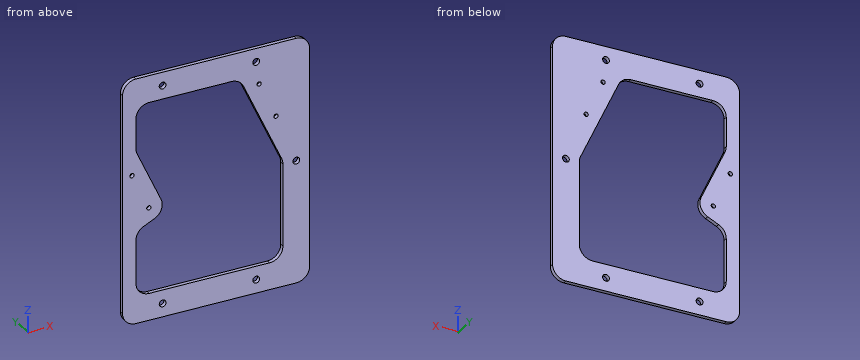
```python
from build123d import *

# Parameters (mm, degrees)
SKETCH_1_W          = 140
SKETCH_1_H          = 182.5
SKETCH_1_R          = 2.55
EXTRUDE_1_DEPTH     = 3
FILLET_1_R          = 10
SKETCH_2_R          = 1.6
CUT_EXTRUDE_1_DEPTH = 116.045914747
CUT_EXTRUDE_2_DEPTH = 116.045914747
FILLET_2_R          = 10


with BuildPart() as part:
    # ｽｹｯﾁ1 → ﾎﾞｽ - 押し出し1 (new body)
    with BuildSketch(Plane(origin=(0, 0, 0), x_dir=(1, 0, 0), z_dir=(0, 1, 0))):
        Rectangle(SKETCH_1_W, SKETCH_1_H)
        with Locations(Location((-40, 81.25, 0), (0, 0, 270))):
            Circle(SKETCH_1_R, mode=Mode.SUBTRACT)
        with Locations(Location((30, 81.25, 0), (0, 0, 270))):
            Circle(SKETCH_1_R, mode=Mode.SUBTRACT)
        with Locations(Location((60, 0, 0), (0, 0, 270))):
            Circle(SKETCH_1_R, mode=Mode.SUBTRACT)
        with Locations(Location((-40, -81.25, 0), (0, 0, 270))):
            Circle(SKETCH_1_R, mode=Mode.SUBTRACT)
        with Locations(Location((30, -81.25, 0), (0, 0, 270))):
            Circle(SKETCH_1_R, mode=Mode.SUBTRACT)
    extrude(amount=EXTRUDE_1_DEPTH)

    # ﾌｨﾚｯﾄ1
    fillet_1_edges = [part.edges().sort_by_distance(p)[0] for p in [
        (70, 1.5, 91.25),
        (-70, 1.5, 91.25),
        (-70, 1.5, -91.25),
        (70, 1.5, -91.25),
    ]]
    fillet(fillet_1_edges, radius=FILLET_1_R)

    # ｽｹｯﾁ2 → ｶｯﾄ - 押し出し1 (cut, through all)
    with BuildSketch(Plane(origin=(0, 3, 0), x_dir=(1, 0, 0), z_dir=(0, 1, 0))):
        with Locations(Location((-50.304962764, 7.366722093, 0), (0, 0, 270))):
            Circle(SKETCH_2_R)
        with Locations(Location((-62.983510616, -19.822511518, 0), (0, 0, 270))):
            Circle(SKETCH_2_R)
        with Locations(Location((44.857354875, -37.008195389, 0), (0, 0, 270))):
            Circle(SKETCH_2_R)
        with Locations(Location((32.178807023, -64.197429, 0), (0, 0, 270))):
            Circle(SKETCH_2_R)
    extrude(amount=-CUT_EXTRUDE_1_DEPTH, mode=Mode.SUBTRACT)

    # ｽｹｯﾁ3 → ｶｯﾄ - 押し出し2 (cut, through all)
    with BuildSketch(Plane(origin=(0, 3, 0), x_dir=(1, 0, 0), z_dir=(0, 1, 0))):
        Polygon((-60, 71.25), (50, 71.25), (50, -2.317741498), (17.856359967, -71.25), (-60, -71.25), (-60, -37.086368186), (-37.015702276, 12.203617346), (-60, 22.921371393), align=None)
    extrude(amount=-CUT_EXTRUDE_2_DEPTH, mode=Mode.SUBTRACT)

    # ﾌｨﾚｯﾄ2
    fillet_2_edges = [part.edges().sort_by_distance(p)[0] for p in [
        (-60, 1.5, -22.921371393),
        (-60, 1.5, -71.25),
        (50, 1.5, -71.25),
        (50, 1.5, 2.317741498),
        (17.856359967, 1.5, 71.25),
        (-60, 1.5, 71.25),
        (-60, 1.5, 37.086368186),
        (-37.015702276, 1.5, -12.203617346),
    ]]
    fillet(fillet_2_edges, radius=FILLET_2_R)


solid = part.part
```
Work out the finished part from the listing and answer in its coordinate system (mm). Give positions to 0.01 mm unless a question says otherwise; leave off trailing zeros. Write each loop counter-clockwise with the first axis right and the second up, starting at its lowest first coordinate (ties: lowest second). Pieces come first, ordered by that corner, then holes. Notation, with made-up numbers: (5, -16) -> (54, -16) arc R22 cw to (54, 23) -> close; hole circle Ø11 at (33.25, 83). An arc over 180 degrees is marked (long way). Write item = value, one per line.
Q1. Flat-ended cylindrical pins translate along their axes: pin 1 Ø2.5 at (x, z) = (32.18, 64.2) entering from -Y; pin 2 Ø6 at (x, z) = (-40, 81.25) entering from -Y. Find the tip coordinate at first contact, or state that the pin passes through.
Computed values:
pin_1 = through
pin_2 = 0
Q2. Section A-A on x = 7 is taken. Determine the outline of the cut face in (y, z), and give its area (3 significant figures).
Computed values:
outline = (0, -91.25) -> (3, -91.25) -> (3, -71.25) -> (0, -71.25) -> close; (0, 71.25) -> (3, 71.25) -> (3, 91.25) -> (0, 91.25) -> close
area = 120 mm^2
Q3. Consider line 1 along X through (y, z) = (1.25, -81.25); line 2 along X through (y, z) = (0.3, 2); line 3 along Z through (x, y) = (-12, 2). Determine where each line is inside the solid, lowest interval first.
Computed values:
line_1 = -70 to -42.55, -37.45 to 27.45, 32.55 to 70
line_2 = -70 to -43.64, 49.82 to 58.42, 61.58 to 70
line_3 = -91.25 to -71.25, 71.25 to 91.25
Q4. Section B-B on y = 1.65 is taken. State how many separate pieces and enclosed holes the cut face has, and give its area (3 significant figures).
Computed values:
separate_pieces = 1
enclosed_holes = 10
area = 11,500 mm^2
